Input: part model. Units: mm. Frame: model coordinates. A direction names the side the tool comes from. Give positions to 0.01 mm unless a question says otherwise; leave off trailing zeros. Loops run counter-clockwise (first coordinate to the right, second up) from the corner with the lowest first, then second, coordinate; pieces in that order, holes last.
Solid Edge part; units mm, degrees
sketch "Sketch1" plane through (0, 0, 0) normal (0, 0, 1) x (1, 0, 0)
  line L0 (-68.5, -40) -> (68.5, -40)
  line L1 (68.5, -40) -> (68.5, 40)
  line L2 (68.5, 40) -> (-68.5, 40)
  line L3 (-68.5, 40) -> (-68.5, -40)
  dimension "D1" = 68.5
  dimension "D2" = 68.5
extrude "Extrusionsausprägung_1" add sketch "Sketch1" along normal mid plane 42.56
sketch "Sketch2" plane through (0, 0, 21.28) normal (0, 0, 1) x (1, 0, 0)
  line L0 (-68.5, -40) -> (11.5, -40)
  line L1 (11.5, -40) -> (11.5, -18)
  line L2 (11.5, -18) -> (-68.5, -18)
  line L3 (-68.5, -18) -> (-68.5, -40)
  dimension "D1" = 11.5
  dimension "D2" = 11.5
extrude "Extrusionsausschnitt_1" cut sketch "Sketch2" against normal blind 56
sketch "Sketch3" plane through (0, 0, 21.28) normal (0, 0, 1) x (1, 0, 0)
  line L0 (-68.5, 40) -> (11.5, 40)
  line L1 (11.5, 40) -> (11.5, 28)
  line L2 (11.5, 28) -> (-68.5, 28)
  line L3 (-68.5, 28) -> (-68.5, 40)
  dimension "D1" = 11.5
  dimension "D2" = 11.5
extrude "Extrusionsausschnitt_2" cut sketch "Sketch3" against normal blind 112
sketch "Sketch4" plane through (-27.5, -18, 0) normal (0, -1, 0) x (1, 0, 0)
  line L0 (-41, 5.72) -> (39, 5.72)
  line L1 (39, 5.72) -> (39, 27.4762)
extrude "Extrusionsausschnitt_3" cut sketch "Sketch4" against normal blind 100 material side at (-28.5, -18, 5.77)
sketch "Sketch5" plane through (40, -40, 0) normal (0, -1, 0) x (1, 0, 0)
  line L0 (-28.5, 21.28) -> (28.5, 21.28)
  line L1 (28.5, 21.28) -> (28.5, -21.28)
  line L2 (28.5, -21.28) -> (-28.5, -21.28)
  line L3 (-28.5, -21.28) -> (-28.5, 21.28)
  dimension "D1" = 28.5
  dimension "D2" = 28.5
extrude "Extrusionsausprägung_11" add sketch "Sketch5" along normal blind 3
sketch "Sketch6" plane through (68.5, 0, 0) normal (1, 0, 0) x (0, 1, 0)
  line L0 (40, 21.28) -> (-10, 21.28)
  line L1 (-10, 21.28) -> (-10, 5.72)
  line L2 (-10, 5.72) -> (40, 5.72)
  line L3 (40, 5.72) -> (40, 21.28)
extrude "Extrusionsausschnitt_4" cut sketch "Sketch6" against normal blind 304
hole "Bohrung_1" at (-64.1, 23.6, 21.28) direction (0, 0, -1) diameter 5.8 depth 50.8
hole "Hole1" at (-64.1, -13.6, 21.28) direction (0, 0, -1) diameter 5.8 depth 50.8
hole "Hole2" at (7.1, -13.6, 21.28) direction (0, 0, -1) diameter 5.8 depth 50.8
hole "Hole3" at (15.9, 35.6, 21.28) direction (0, 0, -1) diameter 5.8 depth 50.8
hole "Hole4" at (15.9, -35.6, 21.28) direction (0, 0, -1) diameter 5.8 depth 50.8
hole "Hole5" at (57.1, -14.4, 21.28) direction (0, 0, -1) diameter 5.8 depth 50.8
hole "Hole6" at (64.1, 35.6, 21.28) direction (0, 0, -1) diameter 5.8 depth 50.8
sketch "Sketch7" plane through (-27.5, -18, -7.78) normal (0, -1, 0) x (1, 0, 0)
  circle A0 centre (-4.11, 13.5) radius 13
extrude "Extrusionsausschnitt_8" cut sketch "Sketch7" against normal blind 60
sketch "Sketch8" plane through (68.5, 0, 0) normal (1, 0, 0) x (0, 1, 0)
  circle A0 centre (-26.91, 21.28) radius 6.5
extrude "Extrusionsausschnitt_9" cut sketch "Sketch8" against normal blind 5.05
sketch "Sketch9" plane through (68.5, 0, 0) normal (1, 0, 0) x (0, 0, -1)
  circle A0 centre (-5.72, 5) radius 10.5
extrude "Extrusionsausschnitt_11" cut sketch "Sketch9" against normal blind 8
sketch "Sketch10" plane through (0, 0, -21.28) normal (0, 0, -1) x (1, 0, 0)
  line L0 (25.5, 15) -> (48, 15)
  line L1 (48, 15) -> (48, -25)
  line L2 (48, -25) -> (25.5, -25)
  line L3 (25.5, -25) -> (25.5, 15)
  dimension "D1" = 25.5
  dimension "D2" = 25.5
  dimension "D3" = 48
extrude "Extrusionsausprägung_8" add sketch "Sketch10" along normal blind 5
fillet "Verrundung_7" radius 1 8 edges at (36.75, 25, -21.28) (25.5, 5, -21.28) (48, 5, -21.28) (36.75, -15, -21.28) (36.75, -15, -26.28) (48, 5, -26.28) (25.5, 5, -26.28) (36.75, 25, -26.28)
sketch "Sketch11" plane through (0, 0, -21.28) normal (0, 0, -1) x (1, 0, 0)
  line L0 (-59.11, -22.11) -> (-4.11, -22.11)
  line L1 (-4.11, -22.11) -> (-4.11, -4.11)
  line L2 (-4.11, -4.11) -> (-59.11, -4.11)
  line L3 (-59.11, -4.11) -> (-59.11, -22.11)
  dimension "D1" = 4.11
  dimension "D2" = 4.11
extrude "Extrusionsausprägung_10" add sketch "Sketch11" along normal blind 5
fillet "Verrundung_14" radius 1 8 edges at (-31.61, 22.11, -21.28) (-4.11, 13.11, -21.28) (-31.61, 4.11, -21.28) (-59.11, 13.11, -21.28) (-31.61, 4.11, -26.28) (-59.11, 13.11, -26.28) (-31.61, 22.11, -26.28) (-4.11, 13.11, -26.28)
sketch "Sketch12" plane through (-55.555, 5, 5.72) normal (0, 0, 1) x (0, -1, 0)
  line L0 (-23, 36.945) -> (-21.29, 36.945)
  line L1 (-21.29, 36.945) -> (-21.29, 35.445)
  line L2 (-21.29, 35.445) -> (-23, 35.445)
  line L3 (-23, 35.445) -> (-23, 36.945)
  line L4 (23, 36.945) -> (21.29, 36.945)
  line L5 (21.29, 36.945) -> (21.29, 35.445)
  line L6 (21.29, 35.445) -> (23, 35.445)
  line L7 (23, 35.445) -> (23, 36.945)
revolve "Rotationsausprägung_1" add sketch "Sketch12" angle 180 about axis through (-31.61, 37.0953, 5.72) along (0, 1, 0)
sketch "Sketch13" plane through (22.945, 11, 5.72) normal (0, 0, 1) x (0, -1, 0)
  line L0 (-10.29, -41.555) -> (-10.29, -26.055)
  line L1 (-10.29, -26.055) -> (3.71, -26.055)
  line L2 (3.71, -26.055) -> (3.71, -34.555)
  line L3 (3.71, -34.555) -> (15.29, -34.555)
  line L4 (15.29, -34.555) -> (22.29, -41.555)
  line L5 (-10.29, -41.555) -> (22.29, -41.555)
  dimension "D1" = 10.29
revolve "RevolvedCutout1" cut sketch "Sketch13" angle 360 about axis through (-31.61, 30.9909, 5.72) along (0, -1, 0)
sketch "Sketch14" plane through (40, -26.5, 21.28) normal (0, 0, 1) x (-1, 0, 0)
  line L0 (8.5, 0.41) -> (8.5, 6.91)
  line L1 (8.5, 6.91) -> (14.8, 6.91)
  line L2 (14.8, 6.91) -> (14.8, 5.91)
  line L3 (14.8, 5.91) -> (17.8, 5.91)
  line L4 (17.8, 5.91) -> (17.8, 0.41)
  line L5 (8.5, 0.41) -> (17.8, 0.41)
  dimension "D1" = 8.5
revolve "RevolvedCutout2" cut sketch "Sketch14" angle 360 about axis through (69.0678, -26.91, 21.28) along (-1, 0, 0)
sketch "Sketch15" plane through (40, -26.5, 21.28) normal (0, 0, 1) x (-1, 0, 0)
  line L0 (8.5, 0.41) -> (8.5, 13.41)
  line L1 (8.5, 13.41) -> (-6.5, 13.41)
  line L2 (-6.5, 13.41) -> (-6.5, 5.91)
  line L3 (-6.5, 5.91) -> (-23.45, 5.91)
  line L4 (-23.45, 5.91) -> (-23.45, 0.41)
  line L5 (-23.45, 0.41) -> (8.5, 0.41)
  dimension "D1" = 8.5
revolve "RevolvedCutout3" cut sketch "Sketch15" angle 360 about axis through (69.1887, -26.91, 21.28) along (-1, 0, 0)
sketch "Sketch16" plane through (24.195, 11, 5.72) normal (0, 0, 1) x (-1, 0, 0)
  line L0 (-27.355, 6) -> (-22.255, 6)
  line L1 (-22.255, 6) -> (-22.255, 18)
  line L2 (-22.255, 18) -> (-27.355, 18)
  line L3 (-27.355, 18) -> (-27.355, 6)
revolve "RevolvedCutout4" cut sketch "Sketch16" angle 360 about axis through (69.5338, 5, 5.72) along (-1, 0, 0)
sketch "Sketch17" plane through (24.195, 11, 5.72) normal (0, 0, 1) x (-1, 0, 0)
  line L0 (-22.255, 6) -> (-22.255, 34.5)
  line L1 (-22.255, 34.5) -> (-7.305, 34.5)
  line L2 (-7.305, 34.5) -> (-7.305, 6)
  line L3 (-7.305, 6) -> (-22.255, 6)
  dimension "D1" = 22.255
revolve "RevolvedCutout5" cut sketch "Sketch17" angle 360 about axis through (68.5, 5, 5.72) along (-1, 0, 0)
sketch "Sketch18" plane through (24.195, 11, 5.72) normal (0, 0, 1) x (-1, 0, 0)
  line L0 (10.145, 6) -> (10.145, 18)
  line L1 (10.145, 18) -> (15.245, 18)
  line L2 (15.245, 18) -> (15.245, 6)
  line L3 (15.245, 6) -> (10.145, 6)
  dimension "D1" = 10.145
revolve "RevolvedCutout6" cut sketch "Sketch18" angle 360 about axis through (68.5, 5, 5.72) along (-1, 0, 0)
sketch "Sketch19" plane through (24.195, 11, 5.72) normal (0, 0, 1) x (-1, 0, 0)
  line L0 (20.145, 6) -> (25.245, 6)
  line L1 (25.245, 6) -> (25.245, 18)
  line L2 (25.245, 18) -> (20.145, 18)
  line L3 (20.145, 18) -> (20.145, 6)
  dimension "D1" = 25.245
revolve "RevolvedCutout7" cut sketch "Sketch19" angle 360 about axis through (68.5, 5, 5.72) along (-1, 0, 0)
sketch "Sketch20" plane through (24.195, 11, 5.72) normal (0, 0, 1) x (-1, 0, 0)
  line L0 (-27.355, 6) -> (-27.355, 16.5)
  line L1 (-27.355, 16.5) -> (-36.305, 16.5)
  line L2 (-36.305, 16.5) -> (-36.305, 6)
  line L3 (-36.305, 6) -> (-27.355, 6)
revolve "RevolvedCutout8" cut sketch "Sketch20" angle 360 about axis through (68.5, 5, 5.72) along (-1, 0, 0)
sketch "Sketch21" plane through (24.195, 11, 5.72) normal (0, 0, 1) x (-1, 0, 0)
  line L0 (-7.305, 6) -> (-7.305, -12)
  line L1 (-7.305, -12) -> (10.145, -4.5)
  line L2 (10.145, -4.5) -> (10.145, 6)
  line L3 (10.145, 6) -> (-7.305, 6)
revolve "RevolvedCutout9" cut sketch "Sketch21" angle 360 about axis through (68.5, 5, 5.72) along (-1, 0, 0)
sketch "Sketch22" plane through (24.195, 11, 5.72) normal (0, 0, 1) x (-1, 0, 0)
  line L0 (15.245, 6) -> (20.145, 6)
  line L1 (20.145, 6) -> (20.145, -4.5)
  line L2 (20.145, -4.5) -> (15.245, -4.5)
  line L3 (15.245, -4.5) -> (15.245, 6)
revolve "RevolvedCutout10" cut sketch "Sketch22" angle 360 about axis through (-1.05, 5, 5.72) along (1, 0, 0)
sketch "Sketch23" plane through (24.195, 11, 5.72) normal (0, 0, 1) x (-1, 0, 0)
  line L0 (25.245, 16.5) -> (29.245, 16.5)
  line L1 (29.245, 16.5) -> (38.245, 13.5)
  line L2 (38.245, 13.5) -> (38.245, 6)
  line L3 (38.245, 6) -> (25.245, 6)
  line L4 (25.245, 6) -> (25.245, 16.5)
  dimension "D1" = 25.245
revolve "RevolvedCutout11" cut sketch "Sketch23" angle 360 about axis through (14.05, 5, 5.72) along (-1, 0, 0)
sketch "Sketch24" plane through (68.5, -1.5, 0) normal (1, 0, 0) x (0, 0, 1)
  line L0 (21.28, 31.41) -> (21.28, 41.5)
  line L1 (21.28, 41.5) -> (-21.28, 41.5)
  line L2 (-21.28, 41.5) -> (-21.28, -41.5)
  line L3 (-21.28, -41.5) -> (5.72, -41.5)
  line L4 (5.72, -41.5) -> (5.72, -17)
  line L5 (5.72, 4) -> (5.72, 8.5)
  line L6 (5.72, 8.5) -> (21.28, 8.5)
  line L7 (21.28, 8.5) -> (21.28, 19.41)
  arc A0 (5.72, 4) -> (5.72, -17) centre (5.72, -6.5) ccw
  arc A1 (21.28, 19.41) -> (21.28, 31.41) centre (21.28, 25.41) cw
extrude "Extrusionsausprägung_13" add sketch "Sketch24" along normal blind 1
properties part number "2" material "Polykarbonat"
(1) Reachability of faces 1 (the flat face through (58, -10, 13)), 2 (the cylindrical face through (1.536, 4.736, -6.277)) from +Z, -Z, +X, -X, +Y, -Y: full face, straight path, thin tool, end or side. Return the list, or none.
Values follow:
face 1: +Z, +X, -X, +Y
face 2: +Z
(2) Ray query, probe 1 along Y at (x, z) = (-64, -2); probe 2 along X at (y, z) = (23.6, -11.75); probe 3 along X at (y, z) = (-25, 12). Return the intervals inside material, ascending.
Values follow:
probe 1: y = -18 to -16.5, -10.7 to 20.7, 26.5 to 28
probe 2: x = -68.5 to -67, -61.2 to 31.5, 46.45 to 69.5
probe 3: x = 11.5 to 31.5, 46.5 to 69.5
(3) Pin query (flat end, axial travel): pin 1 Ø0.9 at (y, z) = (3.5, -23.5) entering from +X; pin 2 Ø1.5 at (x, z) = (-21, -19.5) entering from -Y; pin 3 Ø0.9 at (y, z) = (1, -24) entering from -X; pin 4 Ø5 at (x, y) = (7.1, -13.6) entering from -Z. Return the tip coordinate at first contact, or that it passes through.
Values follow:
pin 1: stops at x = 48
pin 2: stops at y = -18
pin 3: stops at x = 25.5
pin 4: passes through
(4) Cut plane B-B (y = 35.6). Return the cut outline in (x, z).
Values follow:
outline: (11.5, -21.28) - (13, -21.28) - (13, 5.72) - (11.5, 5.72) - close; (18.8, -21.28) - (61.2, -21.28) - (61.2, 5.72) - (18.8, 5.72) - close; (67, -21.28) - (69.5, -21.28) - (69.5, 5.72) - (67, 5.72) - close
(5) Mould query, pull axis X, two halves, no side actions, for faces 3 (the cylindrical face through (28.31, -26.77, 14.78)), 4 (the cylindrical face through (38.87, 4.115, -22.766)), 5 (the flat face through (-28, -18, -8)), 6 (the flat face through (-68.5, 5, -8)). Classes: +X half, -X half, draft (parallel to the pull), parting line (faces both ways), or undercut.
Values follow:
face 3: undercut
face 4: undercut
face 5: draft
face 6: -X half
(6) Cut plane C-C (x = 7.1). Return the cut outline in (y, z), and give its area (3 significant figures).
Values follow:
outline: (-18, -21.28) - (-16.5, -21.28) - (-16.5, 5.72) - (-18, 5.72) - close; (-10.7, -21.28) - (28, -21.28) - (28, 5.72) - (15.5, 5.72) arc R10.5 cw to (-5.5, 5.72) - (-10.7, 5.72) - close
area: 912 mm2
(7) Cut plane A-A (x = 57.1). Return the cut outline in (y, z).
Values follow:
outline: (-43, -21.28) - (-17.3, -21.28) - (-17.3, 21.28) - (-21.41, 21.28) arc R5.5 cw to (-32.41, 21.28) - (-43, 21.28) - close; (-11.5, -21.28) - (40, -21.28) - (40, 5.72) - (15.5, 5.72) arc R10.5 cw to (-5.5, 5.72) - (-10, 5.72) - (-10, 21.28) - (-11.5, 21.28) - close
(8) Cut plane D-D (y = -35). Return the cut outline in (x, z).
Values follow:
outline: (11.5, -21.28) - (13.06, -21.28) - (13.06, 21.28) - (11.5, 21.28) - close; (18.74, -21.28) - (69.5, -21.28) - (69.5, 21.28) - (46.5, 21.28) - (46.5, 11.1) - (31.5, 11.1) - (31.5, 21.28) - (18.74, 21.28) - close
